Source: three-view drawing plus pictorial views. Frame: mm from the lowest corner of the part. A direction names the side the tool comes from. Give positions to 0.01 mm unless a question says otherwise; leave off trailing zeros. Loops run counter-clockwise (first coordinate to the right, second up) from the corner with the lowest first, then second, coordinate; pieces in that order, holes last. Notation, with made-up numbers: (7, -29) - (66, -29) arc R25 cw to (66, -10) - close; hole circle Ø11 at (-13, -38.5). An arc over 180 degrees is marked (long way). Answer in a Markdown table with one row per item.
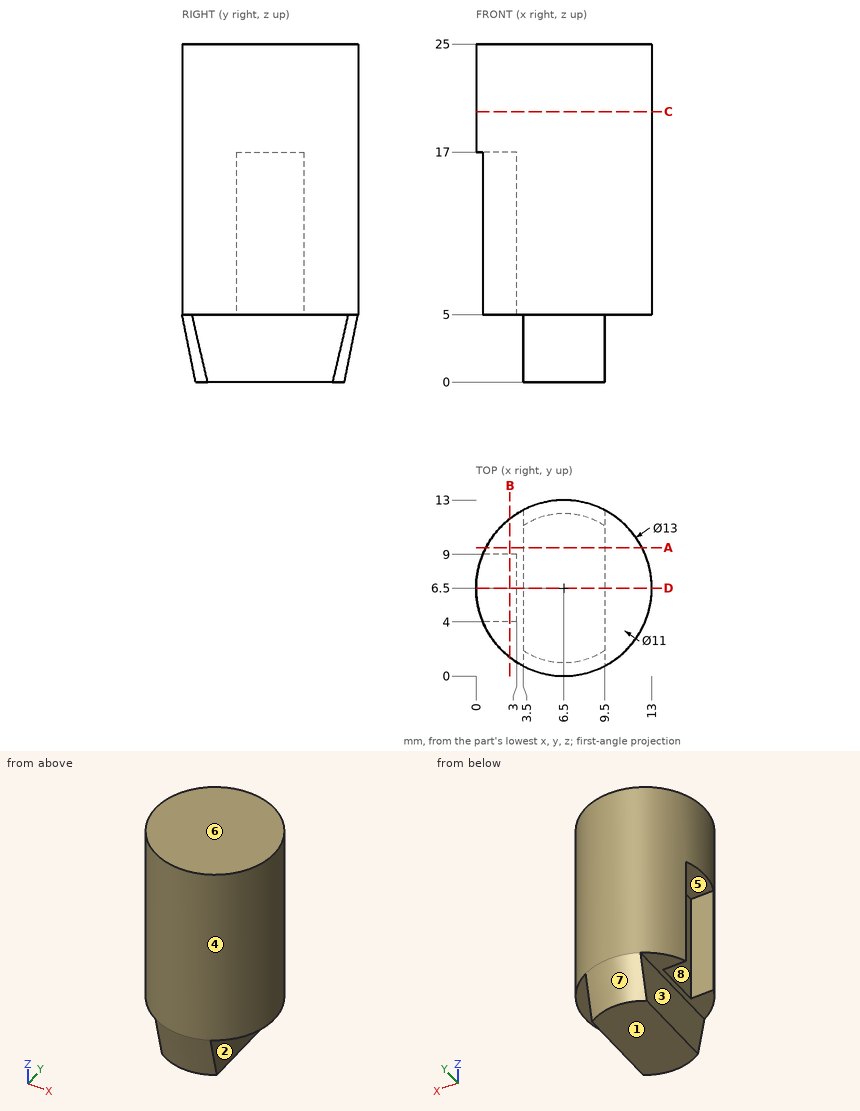
Q1. Cut plane D-D (y = 6.5). Output: boundary loops of the cut face in (x, z), and give its area (3 significant figures).
Check values:
| item | result |
|---|---|
| outline | (0, 17) - (3, 17) - (3, 5) - (3.5, 5) - (3.5, 0) - (9.5, 0) - (9.5, 5) - (13, 5) - (13, 25) - (0, 25) - close |
| area | 254 mm² |
Q2. Draft query along Y for the marked faces 6, 7 and 8. Return one class per face: pulls with the +Y half, pulls with the -Y half, needs draft (parallel to the pull), parting line crosses it, or undercut.
Check values:
| item | result |
|---|---|
| face 6 | needs draft |
| face 7 | pulls with the +Y half |
| face 8 | undercut |
Q3. Cut plane A-A (y = 9.5). Output: boundary loops of the cut face in (x, z).
Check values:
| item | result |
|---|---|
| outline | (0.73, 5) - (3.5, 5) - (3.5, 0) - (9.5, 0) - (9.5, 5) - (12.27, 5) - (12.27, 25) - (0.73, 25) - close |
Q4. Cut plane C-C (z = 20). Output: boundary loops of the cut face in (x, y), and give its area (3 significant figures).
Check values:
| item | result |
|---|---|
| outline | circle Ø13 at (6.5, 6.5) |
| area | 133 mm² |
Q5. Cut plane B-B (x = 2.5). Output: boundary loops of the cut face in (y, z).
Check values:
| item | result |
|---|---|
| outline | (1.38, 5) - (4, 5) - (4, 17) - (9, 17) - (9, 5) - (11.62, 5) - (11.62, 25) - (1.38, 25) - close |
Q6. First-contact query: pin 1 (1.5 mm diameter, centred on y = 8.5, z = 3.5, fed in from +X); pin 2 (1.5 mm diameter, centred on x = 2.5, z = 16.5, fed in from +Y); pin 3 (2 mm diameter, centred on x = 1, z = 11, fed in from -Y). Flat tips, straight axial feed; report the tip coordinate or a pass-through.
Check values:
| item | result |
|---|---|
| pin 1 | x = 9.5 |
| pin 2 | y = 12.13 |
| pin 3 | y = 1.81 |
Q7. Reachability of the marked faces 1, 2, 3, 4 and 5 from +Z, -Z, +X, -X, +Y, -Y: full face, straight path, thin tool, end or side. Return the list, or none.
Check values:
| item | result |
|---|---|
| face 1 | -Z, +X, -X, +Y, -Y |
| face 2 | -Z, +X, +Y, -Y |
| face 3 | -Z, -X, +Y, -Y |
| face 4 | +Z, -Z |
| face 5 | -Z, -X |
Q8. Material intervals for line 1 along X through (y, z) = (6.25, 16.25); line 2 along Z through (x, y) = (11.5, 9.75); line 3 along Y through (x, z) = (12.5, 20.5), sorted ascending.
Check values:
| item | result |
|---|---|
| line 1 | 3 to 13 |
| line 2 | 5 to 25 |
| line 3 | 4 to 9 |
